```python
from build123d import *

# Parameters (mm, degrees)
F0_R     = 12.192
F0_R_2   = 9.789627
F1_DEPTH = 5.08
F2_DEPTH = 2.54
F3_R     = 1.016


with BuildPart() as f1:
    # F0 (on Front) → F1 (new body)
    with BuildSketch(Plane.XZ):
        with Locations((-31.946439, 19.858599)):
            Circle(F0_R)
        with Locations((-31.946439, 19.858599)):
            Circle(F0_R_2, mode=Mode.SUBTRACT)
    extrude(amount=-F1_DEPTH)

    # F0 (on Front) → F2 (join)
    with BuildSketch(Plane.XZ):
        with Locations((-31.946439, 19.858599)):
            Circle(F0_R)
        with Locations((-31.946439, 19.858599)):
            Circle(F0_R_2, mode=Mode.SUBTRACT)
    extrude(amount=F2_DEPTH)

    # F3
    f3_edges = [f1.edges().sort_by_distance(p)[0] for p in [
        (-44.138439, -2.54, 19.858599),
        (-41.736067, -2.54, 19.858599),
        (-41.736067, 5.08, 19.858599),
        (-44.138439, 5.08, 19.858599),
    ]]
    fillet(f3_edges, radius=F3_R)


solid = f1.part
```
Could you check a few things on this model? Use its own coordinates, in mm. Coordinates: 2 decimals unless noted, no trailing zeros. Write each loop counter-clockwise with the first axis right and the second up, starting at its lowest first coordinate (ties: lowest second). Pieces come first, ordered by that corner, then holes. Notation, with made-up numbers: (26.25, 29) -> (67.25, 29) arc R20 ccw to (67.25, 58) -> close; hole circle Ø6 at (28, 77). An arc over 180 degrees is marked (long way). Write item = value, one per line. Start each with the question number.
(1) Will these pins go through, and if not, where does the flat tip stop? pin 1 (5 mm diameter, centred on x = -39.5, z = 19, fed in from +Y); pin 2 (2 mm diameter, centred on x = -40.5, z = 16.5, fed in from -Y).
(2) I need wall thicknesses on line 1 (X direction, y = -1, z = 19.75); line 2 (X direction, y = -1.5, z = 14.75); line 3 (Z direction, x = -30.5, y = 1.5). Which ranges of each line are inside material? Lowest first, please. Write a range as [from, to].
(3) I want a section at B-B (y = 0.5). Please give me the cut outline in (x, z), plus the area to 3 significant figures.
(4) I want a section at A-A (y = 4.5). Please give me the cut outline in (x, z).
Result set:
q1.pin_1 = 4.8
q1.pin_2 = -2.33
q2.line_1 = [-44.14, -41.74], [-22.16, -19.75]
q2.line_2 = [-43.02, -40.3], [-23.6, -20.88]
q2.line_3 = [7.75, 10.18], [29.54, 31.96]
q3.outline = circle Ø24.38 at (-31.95, 19.86); hole circle Ø19.58 at (-31.95, 19.86)
q3.area = 166 mm2
q4.outline = circle Ø24.19 at (-31.95, 19.86); hole circle Ø19.78 at (-31.95, 19.86)
